from build123d import *

# Parameters (mm, degrees)
F1_DEPTH = 5
F2_SIZE  = 4.99999


# Not quite as in the source:
# - a fillet or chamfer is up to 0.001 mm smaller than in the source, because OpenCascade refuses the exact size


with BuildPart() as f1:
    # F0 (on Top) → F1 (new body, symmetric)
    with BuildSketch(Plane.XY):
        Polygon((-5, 7.5), (0, -7.5), (5, 7.5), (5, 16.5857542306), (-5, 16.5857542306), align=None)
    extrude(amount=F1_DEPTH, both=True)

    # F2 (size 5 in the source; OpenCascade refuses exactly that, so slightly less here)
    f2_edges = [f1.edges().sort_by_distance(p)[0] for p in [
        (2.5, 0, -5),
        (-2.5, 0, -5),
        (2.5, 0, 5),
        (-2.5, 0, 5),
    ]]
    chamfer(f2_edges, length=F2_SIZE)


solid = f1.part
Input: part model. Units: mm. Frame: model coordinates. Round coordinates to 2 decimals unless told otherwise and drop trailing zeros. Loops run counter-clockwise (first coordinate to the right, second up) from the corner with the lowest first, then second, coordinate; pieces in that order, holes last. Notation, with made-up numbers: M 50.5,39 L 59.5,39 A29 ccw 59.5,65 Z; hole C 82,37 d6. An arc over 180 degrees is marked long. Answer as CSV lines item,"result". Start each with the question number.
(1) First-contact query: pin 1 (1.5 mm diameter, centred on x = 3.5, y = 1.5, fed in from +Z); pin 2 (2 mm diameter, centred on x = -1.5, y = 1, fed in from +Z). Flat tips, straight axial feed; report the tip coordinate or a pass-through.
(2) Section D-D, the plane y = 13.5. Output: boundary loops of the cut face in (x, z), plus the area to 3 significant figures.
(3) Line query: line 1 (X direction, y = 2.5, z = -1.75); line 2 (X direction, y = 8.5, z = 2.75); line 3 (Z direction, x = 0.75, y = 8). Output: solid intervals per line, ascending. Write a range as [from, to].
(4) Section B-B, the plane z = 2.25. Output: boundary loops of the cut face in (x, y), plus the area to 3 significant figures.
(5) Section A-A, the plane y = 9. Output: boundary loops of the cut face in (x, z).
Values found:
1,pin 1,"stops at z = 0.28"
1,pin 2,"stops at z = 2.26"
2,outline,"M -5,-1.9 L -1.73,-5 L 1.73,-5 L 5,-1.9 L 5,1.9 L 1.73,5 L -1.73,5 L -5,1.9 Z"
2,area,"79.7 mm²"
3,line 1,"x = [-1.49, 1.49]"
3,line 2,"x = [-2.43, 2.43]"
3,line 3,"z = [-4.19, 4.19]"
4,outline,"M -5,14.62 L 0,-0.38 L 5,14.62 L 5,16.59 L -5,16.59 Z"
4,area,"94.7 mm²"
5,outline,"M -5,-0.47 L -0.23,-5 L 0.23,-5 L 5,-0.47 L 5,0.47 L 0.23,5 L -0.23,5 L -5,0.47 Z"
